Verification items for the finished model (mm, model axes). Give positions to 0.01 mm unless a question says otherwise; leave off trailing zeros. Loops run counter-clockwise (first coordinate to the right, second up) from the corner with the lowest first, then second, coordinate; pieces in that order, holes last. Notation, with made-up numbers: M -39,0 L 13,0 A18 ccw 13,14 Z; hole C 19.25,-28.5 d10. An arc over 180 degrees is marked long. Answer in a Markdown table with one row per item.
Autodesk Inventor part; units mm, degrees
ref_plane "YZ Plane" through (0, 0, 0) normal (1, 0, 0) x (0, 1, 0)
ref_plane "XZ Plane" through (0, 0, 0) normal (0, 1, 0) x (-1, 0, 0)
ref_plane "XY Plane" through (0, 0, 0) normal (0, 0, 1) x (1, 0, 0)
sketch "Sketch1" plane through (0, 0, 0) normal (0, 0, 1) x (1, 0, 0)
  line L0 (24.6062, -15.875) -> (-24.6062, -15.875)
  line L1 (-24.6062, -15.875) -> (-24.6062, 15.875)
  line L2 (-24.6062, 15.875) -> (24.6062, 15.875)
  line L3 (24.6062, 15.875) -> (24.6062, -15.875)
  line L4 (24.6062, -15.875) -> (-24.6062, 15.875) construction
  line L5 (-24.6062, -15.875) -> (24.6062, 15.875) construction
  circle A0 centre (24.6062, 15.875) radius 0.7937
  circle A1 centre (-24.6062, 15.875) radius 0.7937
  circle A2 centre (24.6062, -15.875) radius 0.7937
  circle A3 centre (-24.6062, -15.875) radius 0.7937
  line L6 (-24.6062, -15.875) -> (-24.6062, -22.225)
  line L7 (-24.6062, -15.875) -> (-30.9563, -15.875)
  line L8 (-30.9563, -22.225) -> (32.5437, -22.225)
  line L9 (32.5437, -22.225) -> (32.5437, 31.75)
  line L10 (32.5437, 31.75) -> (-30.9563, 31.75)
  line L11 (-30.9563, 31.75) -> (-30.9563, -22.225)
  line L12 (24.6062, 15.875) -> (-12.2237, 15.875)
  line L13 (-30.9563, 31.75) -> (-30.9563, -22.225)
  line L14 (-24.6062, 15.875) -> (12.2237, 15.875)
  line L15 (12.2237, 15.875) -> (12.2237, -20.955)
  line L16 (12.2237, -20.955) -> (-24.6062, -20.955)
  line L17 (-24.6062, -20.955) -> (-24.6062, 15.875)
  circle A4 centre (12.2237, -20.955) radius 0.7937
  line L18 (-24.6062, 15.875) -> (-24.6062, 44.45)
  line L19 (24.6062, -15.875) -> (24.6062, -44.45)
  circle A5 centre (24.6062, -44.45) radius 3.175
  circle A6 centre (-24.6062, 44.45) radius 3.175
  line L20 (33.3375, -50.8) -> (-33.3375, -50.8)
  line L21 (-33.3375, -50.8) -> (-33.3375, 50.8)
  line L22 (-33.3375, 50.8) -> (33.3375, 50.8)
  line L23 (33.3375, 50.8) -> (33.3375, -50.8)
  line L24 (33.3375, -50.8) -> (-33.3375, 50.8) construction
  line L25 (-33.3375, -50.8) -> (33.3375, 50.8) construction
  point P0 (0, 0)
  dimension "d0" = 49.2125
  dimension "d1" = 31.75
  dimension "d2" = 1.5875
  dimension "d5" = 49.2125
  dimension "d8" = 31.75
  dimension "d11" = 6.35
  dimension "d12" = 6.35
  dimension "d13" = 63.5
  dimension "d14" = 53.975
  dimension "d25" = 36.83
  dimension "d26" = 36.83
  dimension "d27" = 1.5875
  dimension "d28" = 28.575
  dimension "d29" = 28.575
  dimension "d30" = 6.35
  dimension "d31" = 6.35
  dimension "d32" = 66.675
  dimension "d33" = 101.6
sketch "Sketch3" plane through (0, 0, 0) normal (0, 0, 1) x (1, 0, 0)
  line L0 (24.6062, -15.875) -> (-24.6062, -15.875)
  line L1 (-24.6062, -15.875) -> (-24.6062, 15.875)
  line L2 (-24.6062, 15.875) -> (24.6062, 15.875)
  line L3 (24.6062, 15.875) -> (24.6062, -15.875)
  line L4 (24.6062, -15.875) -> (-24.6062, 15.875) construction
  line L5 (-24.6062, -15.875) -> (24.6062, 15.875) construction
  circle A0 centre (24.6062, 15.875) radius 0.7937
  circle A1 centre (-24.6062, 15.875) radius 0.7937
  circle A2 centre (24.6062, -15.875) radius 0.7937
  circle A3 centre (-24.6062, -15.875) radius 0.7937
  line L6 (-24.6062, -15.875) -> (-24.6062, -22.225)
  line L7 (-24.6062, -15.875) -> (-30.9563, -15.875)
  line L8 (-30.9563, -22.225) -> (32.5437, -22.225)
  line L9 (32.5437, -22.225) -> (32.5437, 31.75)
  line L10 (32.5437, 31.75) -> (-30.9563, 31.75)
  line L11 (-30.9563, 31.75) -> (-30.9563, -22.225)
  line L12 (24.6062, 15.875) -> (-12.2237, 15.875)
  line L13 (-30.9563, 31.75) -> (-30.9563, -22.225)
  line L14 (-24.6062, 15.875) -> (12.2237, 15.875)
  line L15 (12.2237, 15.875) -> (12.2237, -20.955)
  line L16 (12.2237, -20.955) -> (-24.6062, -20.955)
  line L17 (-24.6062, -20.955) -> (-24.6062, 15.875)
  circle A4 centre (12.2237, -20.955) radius 0.7937
  line L18 (-24.6062, 15.875) -> (-24.6062, 44.45)
  line L19 (24.6062, -15.875) -> (24.6062, -44.45)
  circle A5 centre (24.6062, -44.45) radius 3.175
  circle A6 centre (-24.6062, 44.45) radius 3.175
  line L20 (33.3375, -50.8) -> (-33.3375, -50.8)
  line L21 (-33.3375, -50.8) -> (-33.3375, 50.8)
  line L22 (-33.3375, 50.8) -> (33.3375, 50.8)
  line L23 (33.3375, 50.8) -> (33.3375, -50.8)
  line L24 (33.3375, -50.8) -> (-33.3375, 50.8) construction
  line L25 (-33.3375, -50.8) -> (33.3375, 50.8) construction
  point P0 (0, 0)
  dimension "d34" = 49.2125
  dimension "d35" = 31.75
  dimension "d36" = 1.5875
  dimension "d37" = 49.2125
  dimension "d38" = 31.75
  dimension "d39" = 6.35
  dimension "d40" = 6.35
  dimension "d41" = 63.5
  dimension "d42" = 53.975
  dimension "d43" = 36.83
  dimension "d44" = 36.83
  dimension "d45" = 1.5875
  dimension "d46" = 28.575
  dimension "d47" = 28.575
  dimension "d48" = 6.35
  dimension "d49" = 6.35
  dimension "d50" = 66.675
  dimension "d51" = 101.6
extrude "Extrusion2" add sketch "Sketch1" along normal blind 6.35 contours A3 L6 L0 | A3 L1 A1 L2 L15 L0 | L0 L1 A3 | L0 L15 A4 L16 L6 A3 | L7 A3 L1 | L6 A3 L7 | L15 L2 A0 L3 A2 L0 | L0 A2 L19 L8 L6 L16 A4 L15 | A3 L7 L11 L10 L18 A1 L1 | L6 L8 L11 L7 A3 | A2 L3 L0 | L0 L19 A2 | L2 A1 L18 L10 L9 L8 L19 A2 L3 A0 | A4 L16 L15 | L15 L16 A4 | A1 L18 L1 | L1 L2 A1 | L3 A2 L19 | A0 L3 L2 | L2 L3 A0 | L18 A1 L2 | L20 L21 L22 L23
extrude "Extrusion3" cut sketch "Sketch3" along normal blind 6.35 contours A3 L6 L0 | L0 L1 A3 | L7 A3 L1 | L6 A3 L7 | A2 L3 L0 | L0 L19 A2 | A4 L16 L15 | L15 L16 A4 | A1 L18 L1 | L1 L2 A1 | L3 A2 L19 | A0 L3 L2 | L2 L3 A0 | L18 A1 L2
sketch "Sketch7" plane through (0, 0, 0) normal (0, 0, -1) x (-1, 0, 0)
  circle A0 centre (-24.6062, 15.875) radius 0.7937
  circle A1 centre (-12.2237, -20.955) radius 0.7937
  circle A2 centre (24.6062, -15.875) radius 0.7937
  circle A3 centre (24.6062, 15.875) radius 0.7937
  circle A4 centre (-24.6062, -15.875) radius 0.7937
  line L0 (-21.8566, 15.875) -> (-23.2314, 13.4938)
  line L1 (-23.2314, 13.4938) -> (-25.9811, 13.4938)
  line L2 (-25.9811, 13.4938) -> (-27.3559, 15.875)
  line L3 (-27.3559, 15.875) -> (-25.9811, 18.2562)
  line L4 (-25.9811, 18.2562) -> (-23.2314, 18.2563)
  line L5 (-23.2314, 18.2563) -> (-21.8566, 15.875)
  line L6 (-21.8566, -15.875) -> (-23.2314, -18.2562)
  line L7 (-23.2314, -18.2562) -> (-25.9811, -18.2562)
  line L8 (-25.9811, -18.2562) -> (-27.3559, -15.875)
  line L9 (-27.3559, -15.875) -> (-25.9811, -13.4937)
  line L10 (-25.9811, -13.4937) -> (-23.2314, -13.4937)
  line L11 (-23.2314, -13.4937) -> (-21.8566, -15.875)
  line L12 (26.9875, -15.875) -> (25.7969, -17.9372)
  line L13 (25.7969, -17.9372) -> (23.4156, -17.9372)
  line L14 (23.4156, -17.9372) -> (22.225, -15.875)
  line L15 (22.225, -15.875) -> (23.4156, -13.8128)
  line L16 (23.4156, -13.8128) -> (25.7969, -13.8128)
  line L17 (25.7969, -13.8128) -> (26.9875, -15.875)
  point P0 (0, 0)
  dimension "d118" = 4.7625
  dimension "d119" = 4.7625
  dimension "d120" = 4.7625
extrude "Extrusion4" cut sketch "Sketch7" against normal blind 1.5875 contours L0 L1 L2 L3 L4 L5 | L6 L7 L8 L9 L10 L11 | L12 L13 L14 L15 L16 L17
sketch "Sketch8" plane through (0, 0, 6.35) normal (0, 0, 1) x (1, 0, 0)
  circle A0 centre (12.2237, -20.955) radius 0.7937
  circle A1 centre (12.2237, -20.955) radius 2.3813
  point P0 (0, 0)
  dimension "d123" = 4.7625
extrude "Extrusion5" cut sketch "Sketch8" against normal blind 3.175
sketch "Sketch9" plane through (0, 0, 6.35) normal (0, 0, 1) x (1, 0, 0)
  circle A0 centre (24.6062, -44.45) radius 3.175
  circle A1 centre (-24.6062, 44.45) radius 3.175
  line L0 (-24.6062, 44.45) -> (24.6062, 44.45)
  line L1 (24.6062, 44.45) -> (24.6062, -44.45)
  line L2 (24.6062, -44.45) -> (-24.6062, -44.45)
  line L3 (-24.6062, -44.45) -> (-24.6062, 44.45)
  circle A2 centre (-24.6062, -44.45) radius 3.175
  circle A3 centre (24.6062, 44.45) radius 3.175
  point P0 (0, 0)
  dimension "d126" = 6.35
  dimension "d127" = 6.35
extrude "Extrusion6" cut sketch "Sketch9" against normal blind 6.35 contours A3 L0 L1 | L1 L0 A3 | A2 L3 L2 | L2 L3 A2
properties part number "lidarCamMount" material "Polyethylene, High Density"
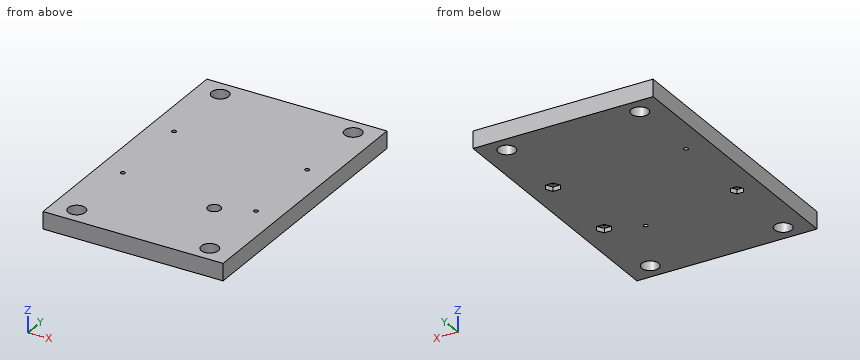
Item 1: Sectioned sample at B-B (y = 45.5). Record the cut outline in (x, z), and give its area (3 significant figures).
Reported:
| item | result |
|---|---|
| outline | M -33.34,0 L -27.6,0 L -27.6,6.35 L -33.34,6.35 Z; M -21.61,0 L 21.61,0 L 21.61,6.35 L -21.61,6.35 Z; M 27.6,0 L 33.34,0 L 33.34,6.35 L 27.6,6.35 Z |
| area | 347 mm^2 |
Item 2: Go/stop test with flat-tipped pins: pin 1 (2 mm diameter, centred on x = 12.22, y = -20.96, fed in from +Z) (3 decimals); pin 2 (2 mm diameter, centred on x = 24.61, y = 15.88, fed in from -Z). Record where each tip stops, or that it passes through.
Reported:
| item | result |
|---|---|
| pin 1 | stops at z = 3.175 |
| pin 2 | stops at z = 1.59 |
Item 3: Sectioned sample at A-A (y = -44.45). Record the cut outline in (x, z), and give its area (3 significant figures).
Reported:
| item | result |
|---|---|
| outline | M -33.34,0 L -27.78,0 L -27.78,6.35 L -33.34,6.35 Z; M -21.43,0 L 21.43,0 L 21.43,6.35 L -21.43,6.35 Z; M 27.78,0 L 33.34,0 L 33.34,6.35 L 27.78,6.35 Z |
| area | 343 mm^2 |
Item 4: Scan lines: L1, parallel to X at y = 44.45, z = 1.5; L2, parallel to Y at x = -23, z = 0.75; L3, parallel to X at y = 46, z = 4.75. Record each from-to range of solid material in increasing order. Write a range as [from, to].
Reported:
| item | result |
|---|---|
| L1 | x = [-33.34, -27.78], [-21.43, 21.43], [27.78, 33.34] |
| L2 | y = [-50.8, -47.19], [-41.71, -17.22], [-14.53, 41.71], [47.19, 50.8] |
| L3 | x = [-33.34, -27.38], [-21.84, 21.84], [27.38, 33.34] |
